Geometry: see drawing. Coordinates: mm, zero at the bounding-box minimum. A direction names the side the tool comes from. Give positions to 0.01 mm unless a question says otherwise; leave off trailing zeros. Loops run counter-clockwise (first coordinate to the right, second up) from the corner with the lowest first, then second, coordinate; pieces in that order, holes last. Notation, with made-up numbers: (32.5, -14.75) -> (80.5, -14.75) arc R18 cw to (80.5, 0.25) -> close; hole circle Ø9 at (-36, 17). An arc over 180 degrees is marked (long way). Return JSON: item names as keys, results as strings. Group by question number.
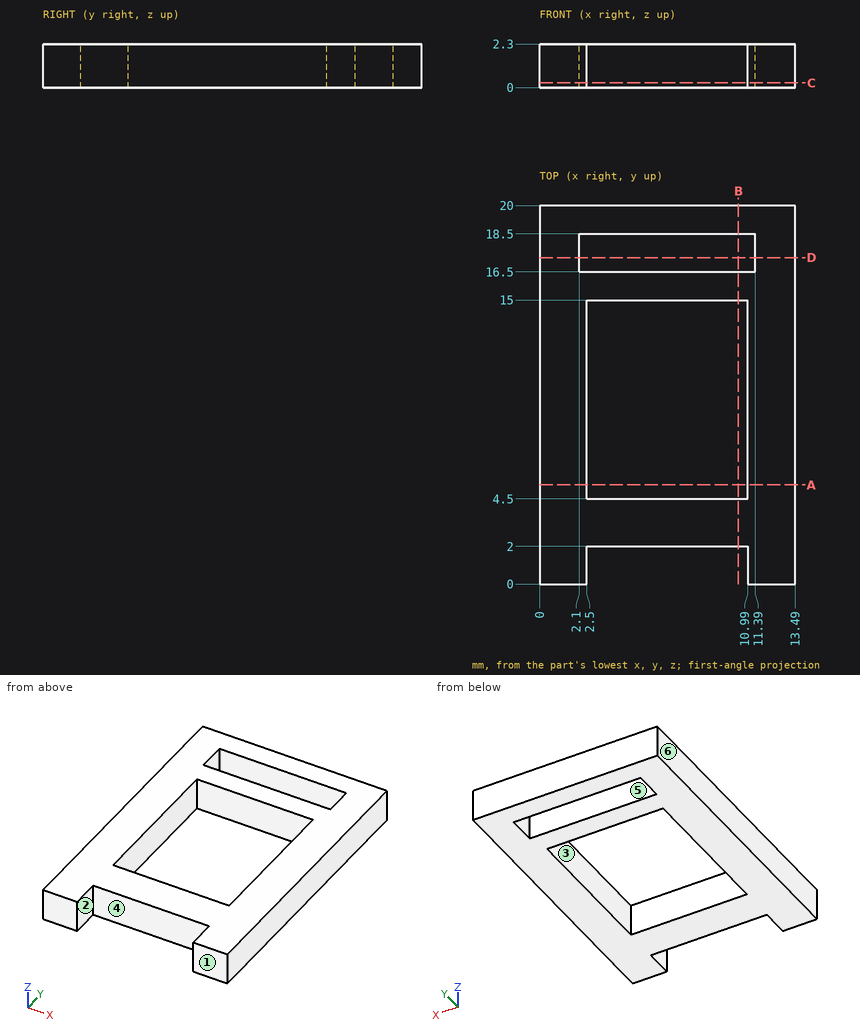
1) Mould query, pull axis Y, two halves, no side actions, for the marked faces 4, 5 and 6. Classes: released by +Y, released by -Y, zero draft, split by the parting line, or undercut.
2) Reachability of the marked faces 1, 2 and 3 from +Z, -Z, +X, -X, +Y, -Y: full face, straight path, thin tool, end or side. Return the list, or none.
3) Contact query for flat-ended pins moving along their axis: P1, Ø1, axis at x = 6, z = 0.5, coming from the -Y side; P2, Ø0.6, axis at y = 1, z = 1.5, coming from the -X side. Output: stop coordinate, or through.
4) Cut plane D-D on y = 17.25. Return loops of the section in (x, z), then the cut area to 3 significant figures.
5) Cut plane C-C on z = 0.25. Return loops of the section in (x, y).
6) Cut plane B-B on x = 10.5. Return loops of the section in (y, z).
7) Material intervals for line 1 (Y direction, x = 7.75, z = 1.8); line 2 (X direction, y = 11.75, z = 1.7); line 3 (X direction, y = 17.75, z = 1.4), sorted ascending.
8) Cut plane A-A on y = 5.25. Return loops of the section in (x, z), then the cut area to 3 significant figures.
Calculated:
{
 "1": {"face 4": "released by -Y", "face 5": "undercut", "face 6": "zero draft"},
 "2": {"face 1": "+Z, -Z, +X, -X, -Y", "face 2": "+Z, -Z, -Y", "face 3": "+Z, -Z"},
 "3": {"P1": "y = 2", "P2": "x = 0"},
 "4": {"outline": "(0, 0) -> (2.1, 0) -> (2.1, 2.3) -> (0, 2.3) -> close; (11.39, 0) -> (13.49, 0) -> (13.49, 2.3) -> (11.39, 2.3) -> close", "area": "9.66 mm2"},
 "5": {"outline": "(0, 0) -> (2.5, 0) -> (2.5, 2) -> (10.99, 2) -> (10.99, 0) -> (13.49, 0) -> (13.49, 20) -> (0, 20) -> close; hole (2.1, 16.5) -> (11.39, 16.5) -> (11.39, 18.5) -> (2.1, 18.5) -> close; hole (2.5, 4.5) -> (10.99, 4.5) -> (10.99, 15) -> (2.5, 15) -> close"},
 "6": {"outline": "(2, 0) -> (4.5, 0) -> (4.5, 2.3) -> (2, 2.3) -> close; (15, 0) -> (16.5, 0) -> (16.5, 2.3) -> (15, 2.3) -> close; (18.5, 0) -> (20, 0) -> (20, 2.3) -> (18.5, 2.3) -> close"},
 "7": {"line 1": "2 to 4.5, 15 to 16.5, 18.5 to 20", "line 2": "0 to 2.5, 10.99 to 13.49", "line 3": "0 to 2.1, 11.39 to 13.49"},
 "8": {"outline": "(0, 0) -> (2.5, 0) -> (2.5, 2.3) -> (0, 2.3) -> close; (10.99, 0) -> (13.49, 0) -> (13.49, 2.3) -> (10.99, 2.3) -> close", "area": "11.5 mm2"}
}
